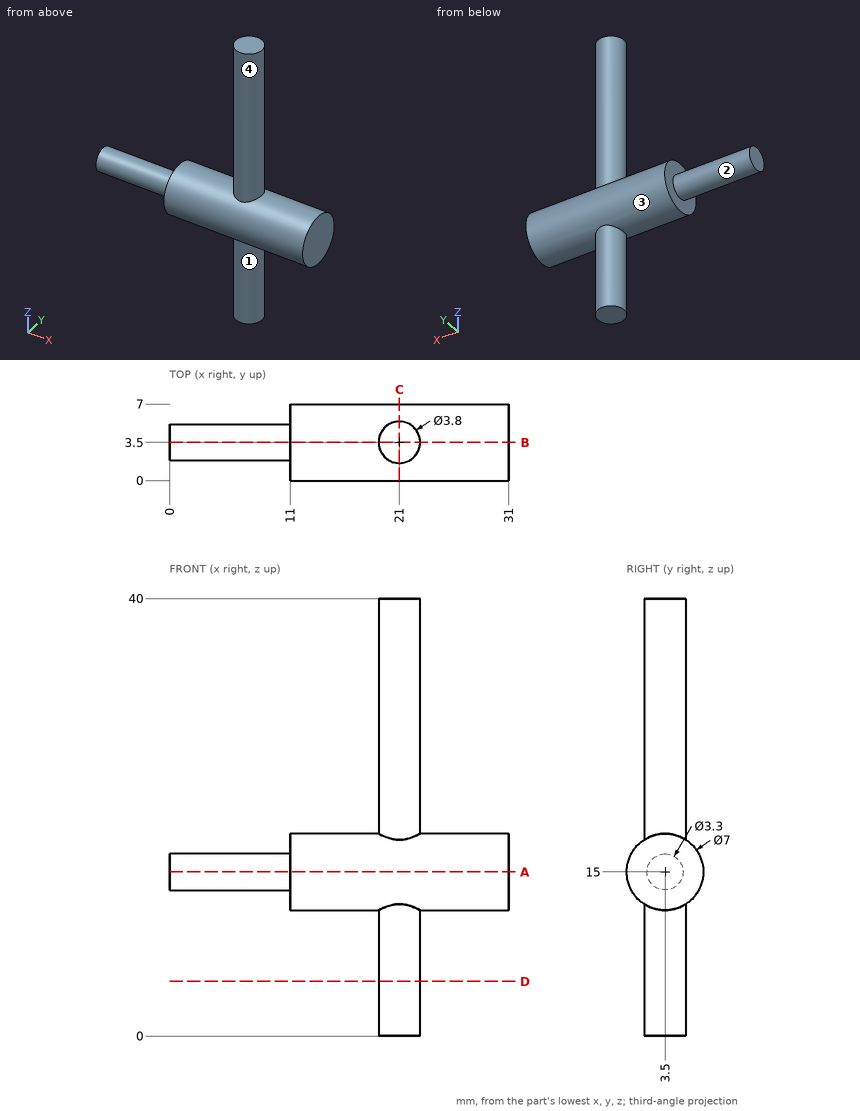
The drawing under review shows one solid part. Ordinate dimensions are in mm from its lowest x, y, z. A direction names the side the tool comes from. Round coordinates to 2 decimals unless told otherwise and drop trailing zeros. Order: outer loops, then holes, each group sorted by start corner. A loop starts at its lowest first (then second) coordinate and runs counter-clockwise, first axis right, second up. Notation, with made-up numbers: (77.5, 44.25) -> (126.5, 44.25) arc R13 ccw to (126.5, 53.25) -> close; hole circle Ø11 at (-1, 72). An arc over 180 degrees is marked (long way). Use a Markdown table: item, result.
Q1. Tool access review of the marked faces 1, 2, 3 and 4: name each direction out of +Z, -Z, +X, -X, +Y, -Y from which nothing blocks a thin tool from reaching the whole face with its end or side.
Values:
| item | result |
|---|---|
| face 1 | -Z |
| face 2 | -X |
| face 3 | none |
| face 4 | +Z |
Q2. We need section B-B on y = 3.5. Write out the cut boundary in (x, z), then the cut area to 3 significant figures.
Values:
| item | result |
|---|---|
| outline | (0, 13.35) -> (11, 13.35) -> (11, 11.5) -> (19.1, 11.5) -> (19.1, 0) -> (22.9, 0) -> (22.9, 11.5) -> (31, 11.5) -> (31, 18.5) -> (22.9, 18.5) -> (22.9, 40) -> (19.1, 40) -> (19.1, 18.5) -> (11, 18.5) -> (11, 16.65) -> (0, 16.65) -> close |
| area | 302 mm^2 |
Q3. We need section C-C on x = 21. Write out the cut boundary in (y, z).
Values:
| item | result |
|---|---|
| outline | (1.6, 0) -> (5.4, 0) -> (5.4, 12.06) arc R3.5 ccw to (5.4, 17.94) -> (5.4, 40) -> (1.6, 40) -> (1.6, 17.94) arc R3.5 ccw to (1.6, 12.06) -> close |
Q4. For line 1 (Z direction, x = 18.5, y = 3.75); line 2 (Y direction, x = 21, z = 37.5); line 3 (X direction, y = 2.25, z = 18), list the stretches that pass through material, from the lowest coordinate up.
Values:
| item | result |
|---|---|
| line 1 | z = 11.51 to 18.49 |
| line 2 | y = 1.6 to 5.4 |
| line 3 | x = 11 to 31 |
Q5. We need section A-A on z = 15. Write out the cut boundary in (x, y), then the cut area to 3 significant figures.
Values:
| item | result |
|---|---|
| outline | (0, 1.85) -> (11, 1.85) -> (11, 0) -> (31, 0) -> (31, 7) -> (11, 7) -> (11, 5.15) -> (0, 5.15) -> close |
| area | 176 mm^2 |
Q6. We need section D-D on z = 5. Write out the cut boundary in (x, y).
Values:
| item | result |
|---|---|
| outline | circle Ø3.8 at (21, 3.5) |
Q7. Clearance check with a flat-ended pin moving along its axis: P1, Ø3, axis at x = 11.5, z = 17.5, coming from the -Y side. State where the tip first meets the part, or that it passes through.
Values:
| item | result |
|---|---|
| P1 | stops at y = 0.15 |
